from build123d import *

# Parameters (mm, degrees)
SKETCH1_R              = 250
BOSS_EXTRUDE1_DEPTH    = 600
CUT_EXTRUDE6_DEPTH     = 600
CUT_EXTRUDE8_START     = -1
CUT_EXTRUDE8_OUTLINE_W = 600
CUT_EXTRUDE8_OUTLINE_H = 174.000412652
CUT_EXTRUDE8_DEPTH     = 1
FILLET2_R              = 120
SKETCH8_R              = 250
CUT_EXTRUDE10_DEPTH    = 120
SKETCH9_R              = 30
CUT_EXTRUDE11_DEPTH    = 1963.141687035


# Read off the part's stored shape, not the designer's step: Cut-Extrude8
with BuildPart() as part:
    # Sketch1 → Boss-Extrude1 (new body)
    with BuildSketch(Plane.XY):
        with BuildLine():
            Line((600, 300), (1800, 300))
            Line((1800, 300), (1800, -300))
            Line((1800, -300), (600, -300))
            ThreePointArc((600, -300), (441.886116992, -325.658350975), (300, -400))
            ThreePointArc((300, -400), (-500, 0), (300, 400))
            ThreePointArc((300, 400), (441.886116992, 325.658350975), (600, 300))
        make_face()
        Circle(SKETCH1_R, mode=Mode.SUBTRACT)
    extrude(amount=BOSS_EXTRUDE1_DEPTH)

    # Sketch2 → Cut-Extrude6 (cut)
    with BuildSketch(Plane(origin=(1800, 0, 0), x_dir=(0, 0, -1), z_dir=(1, 0, 0))):
        Polygon((-180.6, 300), (0, 114), (0, 300), align=None)
        Polygon((-600, -300), (-432.420494682, -300), (-600, -127.409811799), align=None)
        Polygon((-0.445053521, -300), (-0.445053521, -125.999587348), (-179.648136318, -300), align=None)
        Polygon((-606.599587348, 119.845053521), (-606.599587348, 300.445053521), (-420.599587348, 300.445053521), align=None)
    extrude(amount=-CUT_EXTRUDE6_DEPTH, mode=Mode.SUBTRACT)

    # Cut-Extrude8 outline → Cut-Extrude8 (cut)
    with BuildSketch(Plane(origin=(0, 0, 0), x_dir=(-1, 0, 0), z_dir=(0, 0, -1)).offset(CUT_EXTRUDE8_START)):
        with Locations((-1500, -212.999793674)):
            Rectangle(CUT_EXTRUDE8_OUTLINE_W, CUT_EXTRUDE8_OUTLINE_H)
    extrude(amount=CUT_EXTRUDE8_DEPTH, mode=Mode.SUBTRACT)

    # Fillet2
    fillet2_edges = [part.edges().sort_by_distance(p)[0] for p in [
        (1200, 213.126519973, 510.528974059),
        (1200, -213.269211239, 90.324068159),
        (1200, -213.7049059, 516.210247341),
        (1200, 207, 90.3),
    ]]
    fillet(fillet2_edges, radius=FILLET2_R)

    # Sketch8 → Cut-Extrude10 (cut)
    with BuildSketch(Plane(origin=(1800, 0, 0), x_dir=(0, 0, -1), z_dir=(1, 0, 0))):
        with Locations((-300, 0)):
            Circle(SKETCH8_R)
    extrude(amount=-CUT_EXTRUDE10_DEPTH, mode=Mode.SUBTRACT)

    # Sketch9 → Cut-Extrude11 (cut, through all)
    with BuildSketch(Plane(origin=(0, 0, 0), x_dir=(-1, 0, 0), z_dir=(0, 0, -1))):
        with Locations((-1740, 0)):
            Circle(SKETCH9_R)
    extrude(amount=-CUT_EXTRUDE11_DEPTH, mode=Mode.SUBTRACT)


solid = part.part
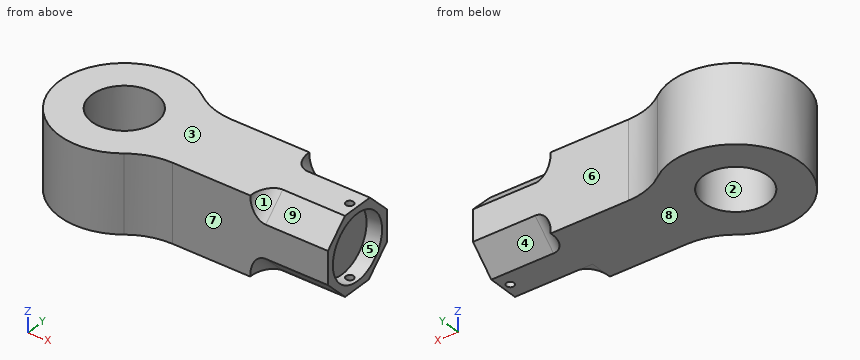
Geometry: final body of the model. Coordinates: model frame, mm. Face numbers are marked on the shaded views. A direction names the side the tool comes from. Coordinates: 2 decimals unless noted, no trailing zeros. Order: outer loops, then holes, each group sorted by start corner. A loop starts at its lowest first (then second) coordinate and runs counter-clockwise, first axis right, second up.
(1) Access query for the marked faces 5, 6, 7, 8 and 9. Directions: +Z, -Z, +X, -X, +Y, -Y. A direction counts if a zero-diameter tool reaches every point of the face in a straight line with its end or side. Return the directions, or none.
(2) Material intervals for probe 1 along Y at (x, z) = (-4, 553); probe 2 along Y at (x, z) = (1773, 300); probe 3 along Z at (x, y) = (1776, 0), sorted ascending.
(3) Section query D-D (x = 1474.5). Return the cut outline in (y, z), plus the area to 3 significant figures.
(4) Section query B-B (z = 300). Return the cut outline in (x, y).
(5) Section query A-A (x = 1740). Return the cut outline in (y, z).
(6) Section query C-C (y = 0). Return the cut outline in (x, z), plus the area to 3 significant figures.
(7) First-contact query: pin 1 (0.8 mm diameter, centred on x = 1649, z = 0.5, fed in from -Y); pin 2 (5 mm diameter, centred on y = -184.5, z = 466, fed in from -X); pin 3 (4 mm diameter, centred on y = -369.5, z = 534, fed in from +X). Flat tips, straight axial feed; report the tip coordinate or a pass-through.
(8) Draft query along Y for the marked faces 1, 2, 3 and 4. Return one class per face: pulls with the +Y half, pulls with the -Y half, needs draft (parallel to the pull), parting line crosses it, or undercut.
Solution:
1. face 5: +X
1. face 6: +Z, -Z, +X, +Y
1. face 7: +Z, -Z, +X, -Y
1. face 8: -Z, +X, -X, +Y, -Y
1. face 9: +Z, +X, -Y
2. probe 1: y = -499.98 to -249.97, 249.97 to 499.98
2. probe 2: y = -300 to -250, 250 to 300
2. probe 3: z = 0 to 50, 550 to 600
3. outline: (-300, 179.65) - (-126.54, 1) - (-126, 1) - (-126, 0) - (114, 0) - (300, 180.6) - (300, 421.06) - (126.25, 600) - (-127.41, 600) - (-300, 432.42) - close
3. area: 298,000 mm2
4. outline: (300, -400) arc R500 cw to (600, -300) - (1800, -300) - (1800, -250) - (1680, -250) - (1680, 250) - (1800, 250) - (1800, 300) - (600, 300) arc R500 cw to (300, 400) arc R500 ccw (long way) to start; hole circle Ø500 at (0, 0)
5. outline: (-300, 179.65) - (-126.54, 1) - (-126, 1) - (-126, 0) - (-30, 0) - (-30, 51.81) arc R250 cw to (-30, 548.19) - (-30, 600) - (-127.41, 600) - (-300, 432.42) - close; (30, 0) - (114, 0) - (300, 180.6) - (300, 421.06) - (126.25, 600) - (30, 600) - (30, 548.19) arc R250 cw to (30, 51.81) - close
6. outline: (-500, 0) - (-250, 0) - (-250, 600) - (-500, 600) - close; (250, 0) - (1710, 0) - (1710, 50) - (1680, 50) - (1680, 550) - (1710, 550) - (1710, 600) - (250, 600) - close; (1770, 0) - (1800, 0) - (1800, 50) - (1770, 50) - close; (1770, 550) - (1800, 550) - (1800, 600) - (1770, 600) - close
6. area: 1,010,000 mm2
7. pin 1: stops at y = -126
7. pin 2: stops at x = -465.7
7. pin 3: stops at x = 349.11
8. face 1: pulls with the -Y half
8. face 2: undercut
8. face 3: needs draft
8. face 4: pulls with the +Y half
